from build123d import *

# Parameters (mm, degrees)
CUT_EXTRUDE1_START = 6.60654
CUT_EXTRUDE1_DEPTH = 2.02616
SKETCH4_R          = 1.833087105
CUT_EXTRUDE2_DEPTH = 1.02616
CUT_EXTRUDE2_DRAFT = -45


with BuildPart() as part:
    # Sketch2 → Revolve1 (revolve)
    with BuildSketch(Plane(origin=(0, 0, 0), x_dir=(0, 0, -1), z_dir=(1, 0, 0))):
        with BuildLine():
            Line((-7.6327, 1.5875), (-7.6327, 2.2225))
            ThreePointArc((-7.6327, 2.2225), (-6.717752118, 3.57733025), (-5.430157143, 4.5847))
            Line((-5.430157143, 4.5847), (-5.0673, 4.5847))
            Line((-5.0673, 4.5847), (-5.0673, 2.413))
            Line((-5.0673, 2.413), (6.83895, 2.413))
            Line((6.83895, 2.413), (7.6327, 1.61925))
            Line((7.6327, 1.61925), (7.6327, 0))
            Line((7.6327, 0), (-5.689996448, 0))
            Line((-5.689996448, 0), (-6.60654, 1.5875))
            Line((-6.60654, 1.5875), (-7.6327, 1.5875))
        make_face()
    revolve(axis=Axis((0, 0, 7.6327), (0, 0, -1)))

    # Sketch3 → Cut-Extrude1 (cut, through all)
    with BuildSketch(Plane.XY.offset(CUT_EXTRUDE1_START)):
        Polygon((0, 1.833087105), (-1.5875, 0.916543552), (-1.5875, -0.916543552), (0, -1.833087105), (1.5875, -0.916543552), (1.5875, 0.916543552), align=None)
    extrude(amount=CUT_EXTRUDE1_DEPTH, mode=Mode.SUBTRACT)


with BuildPart() as cut_extrude2_tool:
    # Sketch4 → Cut-Extrude2 (with draft: the straight prism first)
    with BuildSketch(Plane.XY.offset(7.6327)):
        Circle(SKETCH4_R)
    extrude(amount=-CUT_EXTRUDE2_DEPTH)
    # Cut-Extrude2: the draft: its side faces are tilted about the plane it starts from
    cut_extrude2_sides = [cut_extrude2_tool.faces().sort_by_distance(p)[0] for p in [
        (-1.833087105, 0, 7.11962),
    ]]
    draft(cut_extrude2_sides, Plane.XY.offset(7.6327), CUT_EXTRUDE2_DRAFT)


with BuildPart() as part_1:
    add(part.part)

    # Cut-Extrude2: cut by cut_extrude2_tool
    add(cut_extrude2_tool.part, mode=Mode.SUBTRACT)


solid = part_1.part
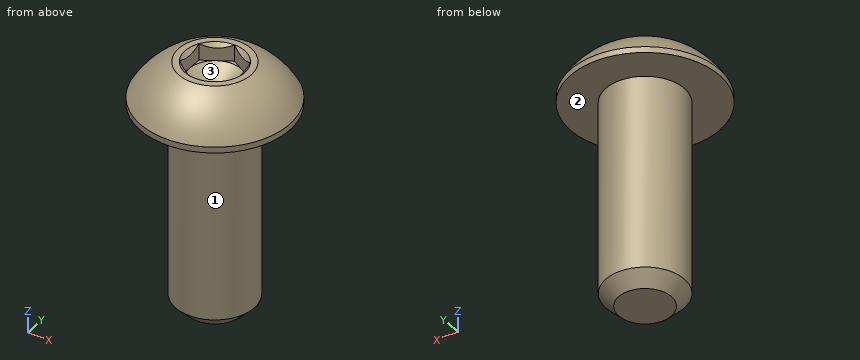
Read the model definition and answer for the solid it produces. Units are mm, in the model's axes. Face numbers are marked on the shaded views. Give positions to 0.01 mm unless a question says otherwise; leave off trailing zeros. Write each loop counter-clockwise with the first axis right and the second up, starting at its lowest first coordinate (ties: lowest second). Pieces come first, ordered by that corner, then holes. Notation, with made-up numbers: (-24.5, 33) - (-12.5, 33) arc R23 ccw to (-12.5, 54) - close; hole circle Ø5 at (-31.75, 69.5). An arc over 180 degrees is marked (long way). Use CSV: the item, a comma, the result in double quotes. Start each with the question number.
(1) Consider line 1 along Z through (x, y) = (3.75, 0.25); line 2 along Z through (x, y) = (-3.25, 1.25); line 3 along X through (y, z) = (1.25, 3). Determine where each line is inside the solid, lowest interval first.
(2) Given P1, Ø0.8, axis at y = -0.5, z = 7, coming from the +X side; P2, Ø2, axis at x = 3, y = 2.5, coming from the +Z side; P3, Ø0.5, axis at x = 0, y = 1.5, coming from the +Z side, each flat-ended and moving along its own axis, determine where each tip first touches the part or whether it passes through.
(3) Find section B-B (y = 4). Give the vertices of the cut face in (x, z).
(4) Determine the mould class of the marked faces 1, 2 and 3 for opening direction Y: +Y half, -Y half, draft (parallel to the pull), parting line (faces both ways), or undercut.
(5) Find section A-A (z = -3.75). Give the vertices of the cut face in (x, y).
Findings below:
1,line 1,"5.07 to 6.54"
1,line 2,"5.07 to 6.8"
1,line 3,"-2.06 to 2.06"
2,P1,"x = 3.67"
2,P2,"z = 7.25"
2,P3,"z = 6.61"
3,outline,"(-2.24, 5.07) - (2.24, 5.07) - (2.24, 5.43) arc R3.39 ccw to (-2.24, 5.43) - close"
4,face 1,"parting line"
4,face 2,"draft"
4,face 3,"undercut"
5,outline,"circle Ø4.83 at (0, 0)"
